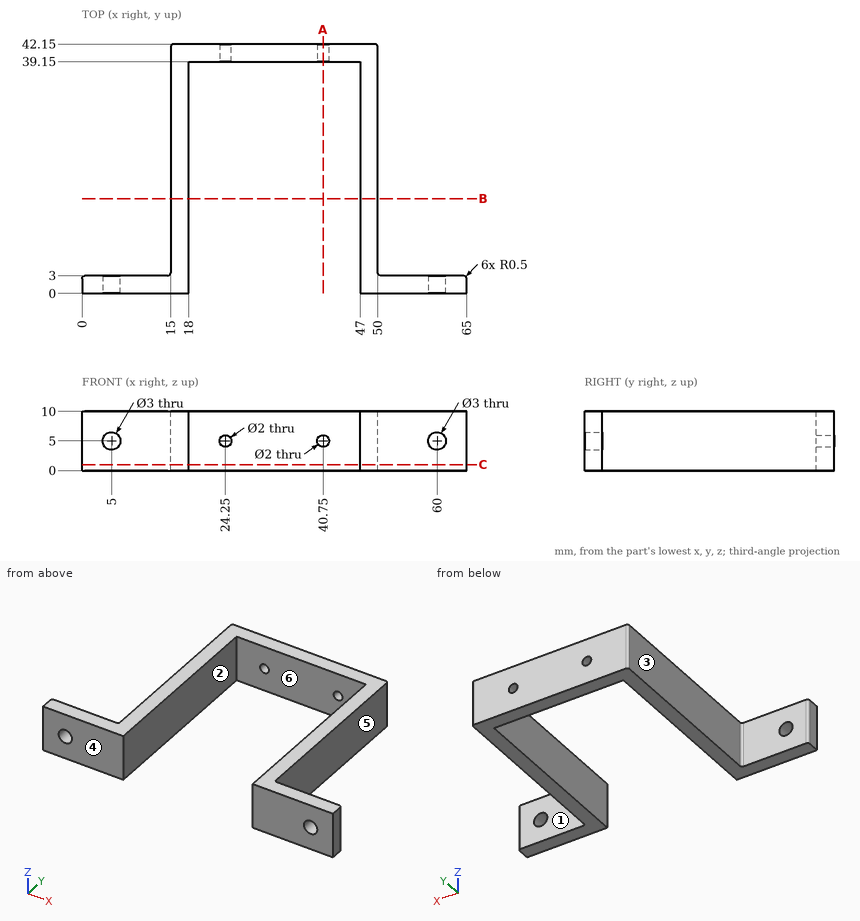
Study the drawing (mm; zero at the part's minimum x, y, z) and answer. A direction names the side the tool comes from. Give positions to 0.01 mm unless a question says otherwise; leave off trailing zeros. Order: outer loops, then holes, each group sorted by start corner. A loop starts at its lowest first (then second) coordinate and runs counter-clockwise, first axis right, second up. Notation, with made-up numbers: (-12, 57) -> (46, 57) arc R35 ccw to (46, 96) -> close; hole circle Ø4 at (-35, -25). An arc over 180 degrees is marked (long way). Write item = value, one per line.
1. A cutting plane is placed at C-C, the plane z = 1. Write down the section's boundary in (x, y).
Numbers:
outline = (0, 0) -> (18, 0) -> (18, 39.15) -> (47, 39.15) -> (47, 0) -> (65, 0) -> (65, 2.5) arc R0.5 ccw to (64.5, 3) -> (50.5, 3) arc R0.5 cw to (50, 3.5) -> (50, 41.65) arc R0.5 ccw to (49.5, 42.15) -> (15.5, 42.15) arc R0.5 ccw to (15, 41.65) -> (15, 3.5) arc R0.5 cw to (14.5, 3) -> (0.5, 3) arc R0.5 ccw to (0, 2.5) -> close
2. A cutting plane is placed at A-A, the plane x = 40.75. Write down the section's boundary in (y, z).
Numbers:
outline = (39.15, 0) -> (42.15, 0) -> (42.15, 4) -> (39.15, 4) -> close; (39.15, 6) -> (42.15, 6) -> (42.15, 10) -> (39.15, 10) -> close
3. For the marked faces 1, 2 and 3, determine the directions among +Z, -Z, +X, -X, +Y, -Y from which every point of the face is accessible in a straight line to the end or side of a thin tool.
Numbers:
face_1 = +Z, -Z, +X, +Y
face_2 = +Z, -Z, -Y
face_3 = +Z, -Z, -X, +Y
4. The mould has two halves that part along X. Classify the marked faces 4, 5 and 6: +X half, -X half, draft (parallel to the pull), parting line (faces both ways), or undercut.
Numbers:
face_4 = draft
face_5 = +X half
face_6 = undercut
5. Given pin 1 (5 mm diameter, centred on y = 16, z = 7, fed in from +X); pin 2 (6 mm diameter, centred on y = 31.5, z = 8, fed in from -X); pin 3 (3 mm diameter, centred on x = 40.75, z = 5, fed in from -Y); pin 4 (4 mm diameter, centred on x = 5, z = 5, fed in from -Y), each flat-ended and moving along its own axis, determine where each tip first touches the part or whether it passes through.
Numbers:
pin_1 = 50
pin_2 = 15
pin_3 = 39.15
pin_4 = 0
6. A cutting plane is placed at B-B, the plane y = 16. Write down the section's boundary in (x, z).
Numbers:
outline = (15, 0) -> (18, 0) -> (18, 10) -> (15, 10) -> close; (47, 0) -> (50, 0) -> (50, 10) -> (47, 10) -> close
7. Straight lines are drawn through the part: line 1 along X through (y, z) = (37, 8.5); line 2 along X through (y, z) = (2, 1.25); line 3 along Z through (x, y) = (60, 0.75). For each, find the intervals that lie inside material, in ascending order.
Numbers:
line_1 = 15 to 18, 47 to 50
line_2 = 0 to 18, 47 to 65
line_3 = 0 to 3.5, 6.5 to 10
